Part model, mm, in its own coordinate system. A direction names the side the tool comes from. Coordinates: 2 decimals unless noted, no trailing zeros. Loops run counter-clockwise (first coordinate to the right, second up) from the corner with the lowest first, then second, coordinate; pieces in that order, holes last. Notation, with made-up numbers: M 80,0 L 120,0 A20 ccw 120,21 Z; hole C -18,16 d2. An arc over 180 degrees is marked long. Use a Markdown table: item, result. Add a question column.
1) Band-saw the part on B-B (x = 10). List the corners of the cut face in (y, z).
2) Band-saw the part on A-A (z = 10). List the corners of the cut face in (x, y).
3) Wall check: probe 1 along X at (y, z) = (-7.25, 11.5); probe 2 along X at (y, z) = (-6.75, 11.75); probe 3 along Z at (x, y) = (-11, -6). Give the ranges that are in metal, low to high. Write a range as from..to.
4) Pin check, flat tips, straight feed: pin 1 Ø5 at (x, z) = (-9, 12) entering from -Y; pin 2 Ø4 at (x, z) = (11, 10) entering from -Y; pin 3 Ø1.5 at (x, z) = (-12, 8) entering from -Y. Stop position of each tip, or through.
5) Band-saw the part on D-D (x = 6.5). List the corners of the cut face in (y, z), plus the area to 3 significant figures.
6) Tool access for faces 1 (the flat face through (-10, -10, 7.8)), 2 (the flat face through (11.7, 0, 7.6)): list every direction of +Z, -Z, +X, -X, +Y, -Y with a clear straight run to the whole face (end or side of a thin tool).
7) Band-saw the part on C-C (y = -12.5). List the corners of the cut face in (x, z).
8) Pull direction Z, two halves, no side cores. Call faces 3 (the flat face through (0, -7, 0)), 4 (the flat face through (0, -7, 20)), 5 (the flat face through (-11.9, 0, 7.6)), 6 (the flat face through (12, -10, 7.8)): released by +Z, released by -Z, zero draft, split by the parting line, or undercut.
from build123d import *

# Parameters (mm, degrees)
PAD_DEPTH       = 20
SKETCH001_R     = 2.25
POCKET_DEPTH    = 15.001
SKETCH002_R     = 5
POCKET001_DEPTH = 5


with BuildPart() as part:
    # Sketch → Pad (new body)
    with BuildSketch(Plane.XY):
        with BuildLine():
            ThreePointArc((-6.05, 0), (0, -6.05), (6.05, 0))
            Line((6.05, 0), (17.5, 0))
            Line((17.5, 0), (17.5, -15))
            Line((17.5, -15), (-17.5, -15))
            Line((-17.5, -15), (-17.5, 0))
            Line((-17.5, 0), (-6.05, 0))
        make_face()
    extrude(amount=PAD_DEPTH)

    # Sketch001 → Pocket (cut, through all)
    with BuildSketch(Plane.XZ.offset(15)):
        with Locations((-11, 10)):
            Circle(SKETCH001_R)
        with Locations((11, 10)):
            Circle(SKETCH001_R)
    extrude(amount=-POCKET_DEPTH, mode=Mode.SUBTRACT)

    # Sketch002 → Pocket001 (cut)
    with BuildSketch(Plane.XZ.offset(15)):
        with Locations((-11.052364, 10)):
            Circle(SKETCH002_R)
        with Locations((10.947636, 10)):
            Circle(SKETCH002_R)
    extrude(amount=-POCKET001_DEPTH, mode=Mode.SUBTRACT)


solid = part.part
Entries:
| question | item | result |
|---|---|---|
| 1 | outline | M -15,0 L 0,0 L 0,7.98 L -10,7.98 L -10,5.09 L -15,5.09 Z; M -15,14.91 L -10,14.91 L -10,12.02 L 0,12.02 L 0,20 L -15,20 Z |
| 2 | outline | M -17.5,-15 L -16.05,-15 L -16.05,-10 L -13.25,-10 L -13.25,0 L -17.5,0 Z; M -8.75,-10 L -6.05,-10 L -6.05,-15 L 5.95,-15 L 5.95,-10 L 8.75,-10 L 8.75,0 L 6.05,0 A6.05 cw -6.05,0 L -8.75,0 Z; M 13.25,-10 L 15.95,-10 L 15.95,-15 L 17.5,-15 L 17.5,0 L 13.25,0 Z |
| 3 | probe 1 | -17.5..-12.68, -9.32..9.32, 12.68..17.5 |
| 3 | probe 2 | -17.5..-12.41, -9.59..9.59, 12.41..17.5 |
| 3 | probe 3 | 0..7.75, 12.25..20 |
| 4 | pin 1 | y = -15 |
| 4 | pin 2 | through |
| 4 | pin 3 | y = -10 |
| 5 | outline | M -15,0 L 0,0 L 0,20 L -15,20 L -15,12.28 L -10,12.28 L -10,7.72 L -15,7.72 Z |
| 5 | area | 277 mm2 |
| 6 | face 1 | -Y |
| 6 | face 2 | +Z, -Z, +X, -X, +Y |
| 7 | outline | M -17.5,0 L 17.5,0 L 17.5,20 L -17.5,20 Z; hole C -11.05,10 d10; hole C 10.95,10 d10 |
| 8 | face 3 | released by -Z |
| 8 | face 4 | released by +Z |
| 8 | face 5 | zero draft |
| 8 | face 6 | undercut |
